Here's how the part is built. I have some questions about the finished solid (model axes, mm). A direction names the side the tool comes from. Round coordinates to 2 decimals unless told otherwise and drop trailing zeros. Loops run counter-clockwise (first coordinate to the right, second up) from the corner with the lowest first, then second, coordinate; pieces in that order, holes last. Notation, with made-up numbers: M 74,3 L 80,3 A24 ccw 80,38 Z; hole C -20,6 d2. An arc over 180 degrees is marked long. Answer as a JSON object with one key per item and string values.
from build123d import *

# Parameters (mm, degrees)
SKETCH1_R           = 4.7625
SKETCH1_R_2         = 2.3241
BOSS_EXTRUDE1_DEPTH = 6.096


with BuildPart() as part:
    # Sketch1 → Boss-Extrude1 (new body)
    with BuildSketch(Plane.XY):
        Polygon((0, 0), (0, 116.205), (119.38, 116.205), (119.38, 0), (119.38, -7.747), (107.442, -7.747), (66.19875, -34.7218), (32.86125, -34.7218), (11.938, -7.747), (0, -7.747), align=None)
        with Locations(Location((59.69, 58.1025, 0), (0, 0, 180))):
            Circle(SKETCH1_R, mode=Mode.SUBTRACT)
        with Locations(Location((39.37, -11.7475, 0), (0, 0, 180))):
            Circle(SKETCH1_R_2, mode=Mode.SUBTRACT)
        with Locations(Location((59.69, -11.7475, 0), (0, 0, 180))):
            Circle(SKETCH1_R_2, mode=Mode.SUBTRACT)
        with Locations(Location((59.69, -24.4475, 0), (0, 0, 180))):
            Circle(SKETCH1_R_2, mode=Mode.SUBTRACT)
        with Locations(Location((39.37, -24.4475, 0), (0, 0, 180))):
            Circle(SKETCH1_R_2, mode=Mode.SUBTRACT)
    extrude(amount=BOSS_EXTRUDE1_DEPTH)


solid = part.part
Item 1: Please list where these lines run through material, in increasing order: probe 1 along Y at (x, z) = (39.37, 4) (3 decimals); probe 2 along Y at (x, z) = (59.69, 5.25) (3 decimals); probe 3 along Y at (x, z) = (109, 3) (3 decimals). Write a range as from..to.
Resolved:
{"probe 1": "-34.722..-26.772, -22.123..-14.072, -9.423..116.205", "probe 2": "-34.722..-26.772, -22.123..-14.072, -9.423..53.34, 62.865..116.205", "probe 3": "-7.747..116.205"}
Item 2: I want a section at D-D, the plane x = 82. Please give me the cut outline in (y, z) (3 decimals), then the cut area to 3 significant figures.
Resolved:
{"outline": "M -24.387,0 L 116.205,0 L 116.205,6.096 L -24.387,6.096 Z", "area": "857 mm²"}
Item 3: I want a section at C-C, the plane z = 4.75. Please give me the cut outline in (x, y) (1 decimal).
Resolved:
{"outline": "M 0,-7.7 L 11.9,-7.7 L 32.9,-34.7 L 66.2,-34.7 L 107.4,-7.7 L 119.4,-7.7 L 119.4,116.2 L 0,116.2 Z; hole C 39.4,-24.4 d4.6; hole C 39.4,-11.7 d4.6; hole C 59.7,58.1 d9.5; hole C 59.7,-24.4 d4.6; hole C 59.7,-11.7 d4.6"}
Item 4: If we mould it in two halves opening along X, with no side actions, what happens to faces 1 (the face through (87.109, -21.046, 3.005)), 2 (the face through (113, -7.747, 3)), 3 (the face through (62, -12, 3))? For each: pulls with the +X half, pulls with the -X half, needs draft (parallel to the pull), parting line crosses it, or undercut.
Resolved:
{"face 1": "pulls with the +X half", "face 2": "needs draft", "face 3": "undercut"}
Item 5: On a 3-axis mill with a long thin cutter (end or side, diameter ignored), from which of +Z, -Z, +X, -X, +Y, -Y can I reach the whole of each face in a straight line? I mean faces 4 (the face through (41.1, -26, 3)), 5 (the face through (6, -7.747, 3)). Say none if no direction works.
Resolved:
{"face 4": "+Z, -Z", "face 5": "+Z, -Z, -X, -Y"}
Item 6: I want a section at A-A, the plane x = 59.69. Please give me the cut outline in (y, z) (3 decimals).
Resolved:
{"outline": "M -34.722,0 L -26.772,0 L -26.772,6.096 L -34.722,6.096 Z; M -22.123,0 L -14.072,0 L -14.072,6.096 L -22.123,6.096 Z; M -9.423,0 L 53.34,0 L 53.34,6.096 L -9.423,6.096 Z; M 62.865,0 L 116.205,0 L 116.205,6.096 L 62.865,6.096 Z"}
Item 7: I want a section at B-B, the plane x = 39.37. Please give me the cut outline in (y, z) (3 decimals).
Resolved:
{"outline": "M -34.722,0 L -26.772,0 L -26.772,6.096 L -34.722,6.096 Z; M -22.123,0 L -14.072,0 L -14.072,6.096 L -22.123,6.096 Z; M -9.423,0 L 116.205,0 L 116.205,6.096 L -9.423,6.096 Z"}
